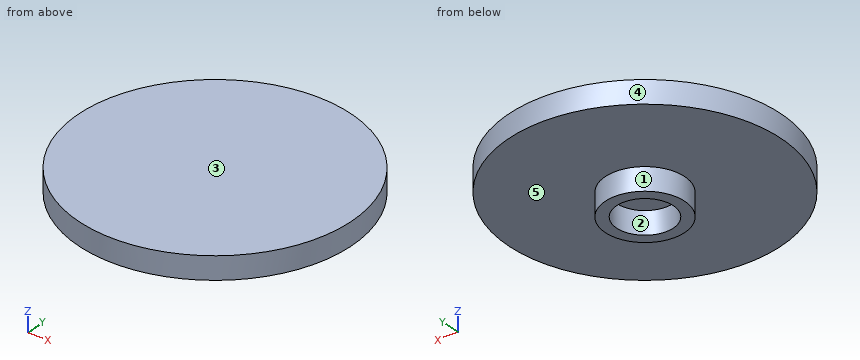
Autodesk Fusion 360 part; units mm, degrees
sketch "Sketch1" plane through (0, 0, 0) normal (0, 0, 1) x (1, 0, 0)
  circle A0 centre (0, 0) radius 12
  dimension "d1" = 24
extrude "Extrude1" add sketch "Sketch1" along normal blind 2
sketch "Sketch2" plane through (0, 0, 0) normal (0, 0, -1) x (1, 0, 0)
  circle A0 centre (0, 0) radius 12
  circle A1 centre (0, 0) radius 2.5
  circle A2 centre (0, 0) radius 3.5
  dimension "d4" = 5
  dimension "d5" = 7
extrude "Extrude2" add sketch "Sketch2" along normal blind 2 contours A2
Build history of the part. All positions in model axes, mm. Face numbers are marked on the shaded views. A direction names the side the tool comes from. Round coordinates to 2 decimals unless told otherwise and drop trailing zeros. Loops run counter-clockwise (first coordinate to the right, second up) from the corner with the lowest first, then second, coordinate; pieces in that order, holes last.
Item 1: Drill centre lines: line 1 along X through (y, z) = (0, -1); line 2 along Z through (x, y) = (8.25, -4.75). Where is each one in solid material? Low to high.
Item 2: Pin check, flat tip, straight feed: P1, Ø1.5, axis at x = 6.5, y = -1.5, coming from the -Z side. Stop position of the tip, or through.
Item 3: Two-plate mould, pull along X, no slides. Class the marked faces 1, 2 and 3: released by +X, released by -X, zero draft, split by the parting line, or undercut.
Item 4: Which spindle directions (+Z, -Z, +X, -X, +Y, -Y) get a long thin tool onto all of the face, cutting with end or side? Do the marked faces 4 and 5. Say none if no direction does.
Item 5: Saw through at D-D (x = -5.75). List the corners of the cut face in (y, z).
Item 6: Saw through at A-A (x = 0). List the corners of the cut face in (y, z), then the cut area to 3 significant figures.
Item 7: Saw through at C-C (z = -0.8). List the corners of the cut face in (x, y).
Worked answers:
1. line 1: x = -3.5 to -2.5, 2.5 to 3.5
1. line 2: z = 0 to 2
2. P1: stops at z = 0
3. face 1: split by the parting line
3. face 2: undercut
3. face 3: zero draft
4. face 4: +Z, -Z
4. face 5: -Z
5. outline: (-10.53, 0) - (10.53, 0) - (10.53, 2) - (-10.53, 2) - close
6. outline: (-12, 0) - (-3.5, 0) - (-3.5, -2) - (-2.5, -2) - (-2.5, 0) - (2.5, 0) - (2.5, -2) - (3.5, -2) - (3.5, 0) - (12, 0) - (12, 2) - (-12, 2) - close
6. area: 52.0 mm2
7. outline: circle Ø7 at (0, 0); hole circle Ø5 at (0, 0)
